Could you check a few things on this model? Use its own coordinates, in mm. Coordinates: 2 decimals unless noted, no trailing zeros. Order: outer loops, then holes, each group sorted by start corner. A loop starts at its lowest first (then second) coordinate and runs counter-clockwise, first axis right, second up. Notation, with made-up numbers: (-25, -24) -> (7, -24) arc R13 cw to (7, -17) -> close; hole circle Ø8 at (-6.75, 43). An arc over 180 degrees is marked (long way). Put each result on its own line as item: value. Start each with the question number.
Q1. Will these pins go through, and if not, where does the flat tip stop? pin 1 (4 mm diameter, centred on x = -115, y = 8, fed in from +Z); pin 2 (1 mm diameter, centred on y = 8, z = -61.5, fed in from -X); pin 3 (14.5 mm diameter, centred on x = -131.57, z = -11.83, fed in from +Y).
Q2. Please list where these lines run through material, in increasing order: line 1 along X through (y, z) = (3, -6); line 2 along Z through (x, y) = (-138, 3.25); line 3 along X through (y, z) = (6, -106).
Q3. If we section it at B-B (z = -87): Please give me the cut outline in (x, y) (3 decimals), and give its area (3 significant figures).
Q4. If we section it at C-C (x = 27): Please give me the cut outline in (y, z) (3 decimals), and give its area (3 significant figures).
Q5. If we section it at A-A (x = -73.5): Please give me the cut outline in (y, z) (3 decimals).
Q6. If we section it at D-D (y = 7): Count the separate pieces of the cut face and the enclosed holes in it, and give its area (3 significant figures).
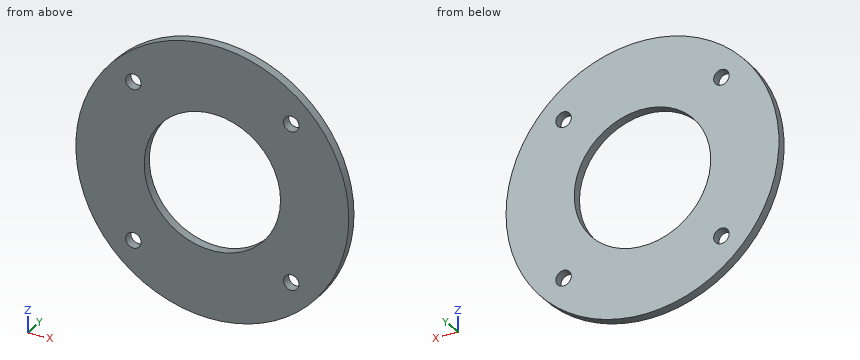
from build123d import *

# Parameters (mm, degrees)
SKETCH1_R           = 139.7
SKETCH1_R_2         = 69.85
SKETCH1_R_3         = 7.9375
BOSS_EXTRUDE1_DEPTH = 9.525


with BuildPart() as part:
    # Sketch1 → Boss-Extrude1 (new body)
    with BuildSketch(Plane(origin=(0, 0, 0), x_dir=(1, 0, 0), z_dir=(0, 1, 0))):
        with Locations((-50.749179719, 92.652131738)):
            Circle(SKETCH1_R)
        with Locations((-50.749179719, 92.652131738)):
            Circle(SKETCH1_R_2, mode=Mode.SUBTRACT)
        with Locations((-131.571484808, 173.474436827)):
            Circle(SKETCH1_R_3, mode=Mode.SUBTRACT)
        with Locations((-131.571484808, 11.829826648)):
            Circle(SKETCH1_R_3, mode=Mode.SUBTRACT)
        with Locations((30.073125371, 11.829826648)):
            Circle(SKETCH1_R_3, mode=Mode.SUBTRACT)
        with Locations((30.073125371, 173.474436827)):
            Circle(SKETCH1_R_3, mode=Mode.SUBTRACT)
    extrude(amount=BOSS_EXTRUDE1_DEPTH)


solid = part.part
The answers:
1. pin 1: z = 32.41
1. pin 2: x = -187.04
1. pin 3: through
2. line 1: -160.33 to -136.96, -126.18 to 24.69, 35.46 to 58.83
2. line 2: -201.75 to -178.13, -168.82 to -16.49, -7.17 to 16.45
2. line 3: -189.81 to -119.31, 17.81 to 88.31
3. outline: (-190.335, 0) -> (-120.37, 0) -> (-120.37, 9.525) -> (-190.335, 9.525) -> close; (18.872, 0) -> (88.836, 0) -> (88.836, 9.525) -> (18.872, 9.525) -> close
3. area: 1,330 mm^2
4. outline: (0, -208.717) -> (9.525, -208.717) -> (9.525, -180.793) -> (0, -180.793) -> close; (0, -166.156) -> (9.525, -166.156) -> (9.525, -19.148) -> (0, -19.148) -> close; (0, -4.511) -> (9.525, -4.511) -> (9.525, 23.413) -> (0, 23.413) -> close
4. area: 1,930 mm^2
5. outline: (0, -230.487) -> (9.525, -230.487) -> (9.525, -158.693) -> (0, -158.693) -> close; (0, -26.611) -> (9.525, -26.611) -> (9.525, 45.183) -> (0, 45.183) -> close
6. separate pieces: 1
6. enclosed holes: 5
6. area: 45,200 mm^2
